Print and shaded views of the part. All mm, measured from the part's lowest x, y and z. A direction names the side the tool comes from. Round coordinates to 2 decimals unless told otherwise and drop trailing zeros. Write each loop counter-clockwise with the first axis right and the second up, starting at its lowest first coordinate (ties: lowest second). Pieces come first, ordered by that corner, then holes.
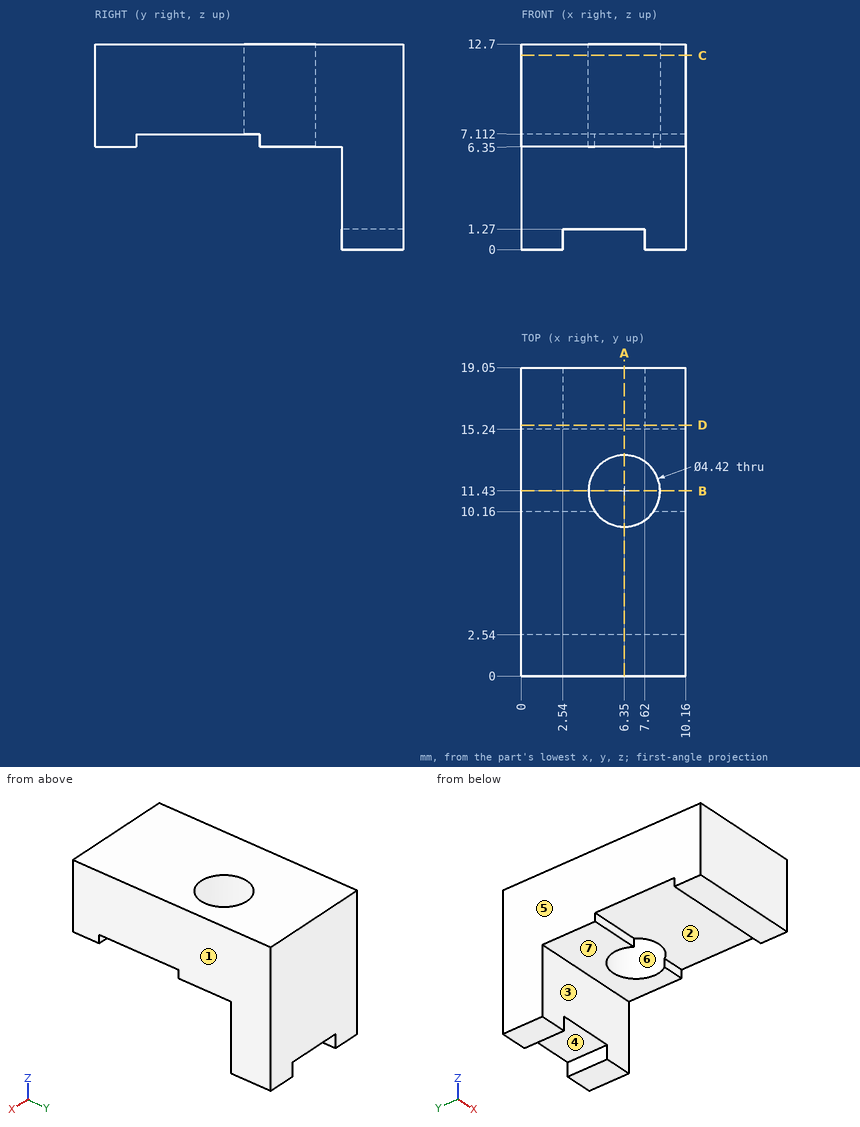
1) Wall check: L1, parallel to X at y = 11.43, z = 9.5; L2, parallel to Y at x = 6.35, z = 11; L3, parallel to Y at x = 5.5, z = 3. Give the ranges that are in metal, low to high.
Results:
L1: x = 0 to 4.14, 8.56 to 10.16
L2: y = 0 to 9.22, 13.64 to 19.05
L3: y = 15.24 to 19.05
2) Which spindle directions (+Z, -Z, +X, -X, +Y, -Y) get a long thin tool onto all of the face, cutting with end or side? Do the marked faces 1, 2 and 3. Say none if no direction does.
Results:
face 1: +Z, -Z, +X, +Y, -Y
face 2: -Z, +X, -X
face 3: -Z, +X, -X, -Y
3) Slice it at A-A (x = 6.35). Write the cut outline in (y, z).
Results:
outline: (0, 6.35) - (2.54, 6.35) - (2.54, 7.11) - (9.22, 7.11) - (9.22, 12.7) - (0, 12.7) - close; (13.64, 6.35) - (15.24, 6.35) - (15.24, 1.27) - (19.05, 1.27) - (19.05, 12.7) - (13.64, 12.7) - close
4) Mould opens along X. For the marked faces 4, 5, 6 and 7 say: released by +X, released by -X, zero draft, split by the parting line, or undercut.
Results:
face 4: undercut
face 5: released by -X
face 6: undercut
face 7: zero draft
5) Pin check, flat tips, straight feed: pin 1 Ø1.3 at (x, y) = (3.5, 1.5) entering from -Z; pin 2 Ø1.5 at (x, y) = (9, 5.5) entering from -Z; pin 3 Ø5 at (x, z) = (5.5, 2) entering from -Y. Stop position of each tip, or through.
Results:
pin 1: stops at z = 6.35
pin 2: stops at z = 7.11
pin 3: stops at y = 15.24
6) Slice it at B-B (y = 11.43). Write the cut outline in (x, z).
Results:
outline: (0, 6.35) - (4.14, 6.35) - (4.14, 12.7) - (0, 12.7) - close; (8.56, 6.35) - (10.16, 6.35) - (10.16, 12.7) - (8.56, 12.7) - close
7) Slice it at D-D (y = 15.5). Write the cut outline in (x, z).
Results:
outline: (0, 0) - (2.54, 0) - (2.54, 1.27) - (7.62, 1.27) - (7.62, 0) - (10.16, 0) - (10.16, 12.7) - (0, 12.7) - close
8) Slice it at C-C (z = 12). Write the cut outline in (x, y).
Results:
outline: (0, 0) - (10.16, 0) - (10.16, 19.05) - (0, 19.05) - close; hole circle Ø4.42 at (6.35, 11.43)
